Input: part model. Units: mm. Frame: model coordinates. A direction names the side the tool comes from. Coordinates: 2 decimals unless noted, no trailing zeros. Write each loop counter-clockwise with the first axis right and the second up, starting at its lowest first coordinate (ties: lowest second). Pieces come first, ordered by that corner, then holes. Notation, with made-up numbers: M 34.25,7 L 41.25,7 A10 cw 41.25,19 Z; hole C -21.5,32.25 d7. An arc over 180 degrees is marked long. Use one line per item in the form item = value.
from build123d import *

# Parameters (mm, degrees)
SKETCH_R     = 4.25
PAD_DEPTH    = 5
POCKET_DEPTH = 2.5
SKETCH002_R  = 2.5
PAD001_DEPTH = 45


with BuildPart() as part:
    # Sketch → Pad (new body)
    with BuildSketch(Plane.XY):
        Circle(SKETCH_R)
    extrude(amount=PAD_DEPTH)

    # Sketch001 → Pocket (cut)
    with BuildSketch(Plane.XY.offset(5)):
        Polygon((0, -2.309401), (2, -1.154701), (2, 1.154701), (0, 2.309401), (-2, 1.154701), (-2, -1.154701), align=None)
    extrude(amount=-POCKET_DEPTH, mode=Mode.SUBTRACT)

    # Sketch002 → Pad001 (join)
    with BuildSketch(Plane.XY):
        Circle(SKETCH002_R)
    extrude(amount=-PAD001_DEPTH)


solid = part.part
(1) Set-up query: faces 1 (the flat face through (1, -2, 5)), 2 (the flat face through (2, -2, 0)), 3 (the flat face through (-2, 0, 4)). Return all of +Z, -Z, +X, -X, +Y, -Y with unobstructed straight access to the full face (end or side cutting, diameter ignored); none if empty.
Computed:
face_1 = +Z, +X, -X, +Y, -Y
face_2 = -Z
face_3 = +Z
(2) Section query C-C on z = -30. Return the cut outline in (x, y), plus the area to 3 significant figures.
Computed:
outline = C 0,0 d5
area = 19.6 mm^2
(3) Section query B-B on x = 1. Return the cut outline in (y, z).
Computed:
outline = M -4.13,0 L -2.29,0 L -2.29,-45 L 2.29,-45 L 2.29,0 L 4.13,0 L 4.13,5 L 1.73,5 L 1.73,2.5 L -1.73,2.5 L -1.73,5 L -4.13,5 Z
(4) Section query D-D on x = -3. Return the cut outline in (y, z), plus the area to 3 significant figures.
Computed:
outline = M -3.01,0 L 3.01,0 L 3.01,5 L -3.01,5 Z
area = 30.1 mm^2
(5) First-contact query: pin 1 Ø2 at (y, z) = (-0.5, -38.5) entering from +X; pin 2 Ø5 at (y, z) = (1.5, -38) entering from -X; pin 3 Ø1 at (y, z) = (2, -31.5) entering from -X; pin 4 Ø4.5 at (x, y) = (0.5, 1) entering from +Z. Flat tips, straight axial feed; report the tip coordinate or a pass-through.
Computed:
pin_1 = 2.5
pin_2 = -2.5
pin_3 = -2
pin_4 = 5
(6) Section query A-A on y = 0. Return the cut outline in (x, z), plus the area to 4 significant figures.
Computed:
outline = M -4.25,0 L -2.5,0 L -2.5,-45 L 2.5,-45 L 2.5,0 L 4.25,0 L 4.25,5 L 2,5 L 2,2.5 L -2,2.5 L -2,5 L -4.25,5 Z
area = 257.5 mm^2
(7) Pull-direction query (X, two-part tool) for faces 4 (the cylindrical face through (-0.54, -2.44, -22.18)), 5 (the flat face through (0, 0, -45)), 6 (the flat face through (-0.99, 1.74, 3.77)); classes: pulls with the +X half, pulls with the -X half, needs draft (parallel to the pull), parting line crosses it, or undercut.
Computed:
face_4 = parting line crosses it
face_5 = needs draft
face_6 = undercut
(8) Line query: probe 1 along Z at (x, y) = (1, 0); probe 2 along Z at (x, y) = (-1.5, 3.75); probe 3 along X at (y, z) = (1.5, -36). Output: solid intervals per line, ascending.
Computed:
probe_1 = -45 to 2.5
probe_2 = 0 to 5
probe_3 = -2 to 2
